Input: dimensioned drawing with shaded views. Units: mm. Origin: part minimum x, y, z. Round coordinates to 2 decimals unless told otherwise and drop trailing zeros. Order: outer loops, then holes, each group sorted by start corner. A loop starts at its lowest first (then second) coordinate and runs counter-clockwise, first axis right, second up. Notation, with made-up numbers: M 17,-8 L 56,-8 A24 ccw 56,23 Z; hole C 80.25,21.25 d9. An arc over 180 degrees is marked long. Put each result on its own line as item: value. Start each with the question number.
1) Section B-B, the plane y = 5.75. Return loops of the section in (x, z) (3 decimals).
2) First-contact query: P1, Ø3, axis at x = 2.5, z = 2.75, coming from the +Y side; P2, Ø5, axis at y = 12, z = 11, coming from the +X side; P3, Ø5, axis at x = 55.5, y = 10, coming from the -Z side. Flat tips, straight axial feed; report the tip coordinate or a pass-through.
3) Section A-A, the plane z = 9. Return loops of the section in (x, y) (3 decimals), then the cut area to 3 significant figures.
4) Section C-C, the plane x = 2.5. Return loops of the section in (y, z) (3 decimals).
5) Material intervals for probe 1 along X at (y, z) = (0.5, 2.75) (3 decimals); probe 2 along Z at (x, y) = (46.5, 0.95) (3 decimals); probe 3 along Y at (x, z) = (31.5, 6), sorted ascending. Write a range as [from, to].
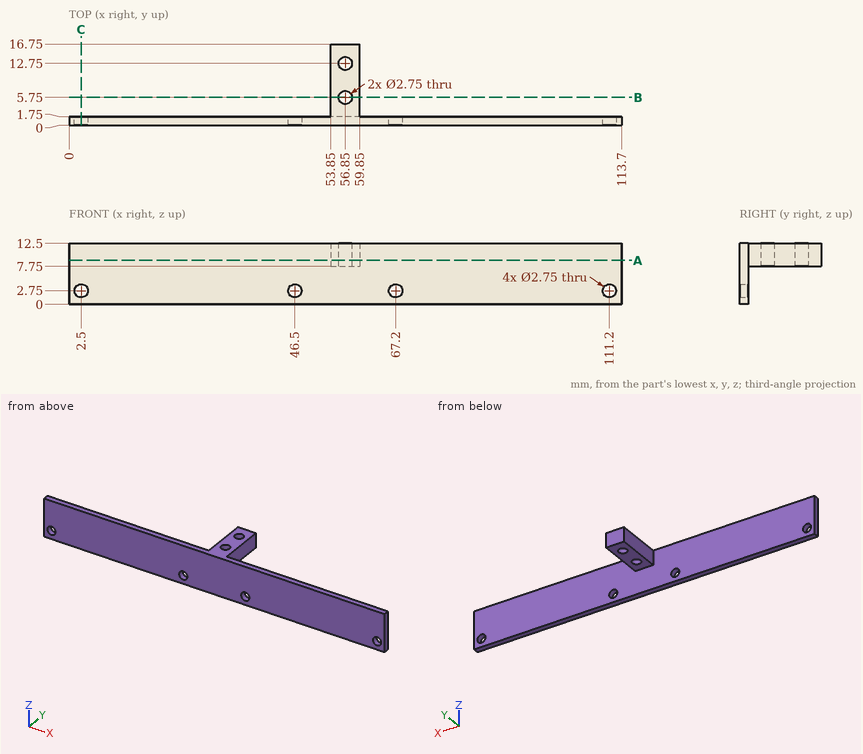
Result sheet:
1. outline: M 53.85,7.75 L 55.475,7.75 L 55.475,12.5 L 53.85,12.5 Z; M 58.225,7.75 L 59.85,7.75 L 59.85,12.5 L 58.225,12.5 Z
2. P1: stops at y = 1.75
2. P2: stops at x = 59.85
2. P3: stops at z = 7.75
3. outline: M 0,0 L 113.7,0 L 113.7,1.75 L 59.85,1.75 L 59.85,16.75 L 53.85,16.75 L 53.85,1.75 L 0,1.75 Z; hole C 56.85,5.75 d2.75; hole C 56.85,12.75 d2.75
3. area: 277 mm2
4. outline: M 0,0 L 1.75,0 L 1.75,1.375 L 0,1.375 Z; M 0,4.125 L 1.75,4.125 L 1.75,12.5 L 0,12.5 Z
5. probe 1: x = [0, 1.125], [3.875, 45.125], [47.875, 65.825], [68.575, 109.825], [112.575, 113.7]
5. probe 2: z = [0, 1.375], [4.125, 12.5]
5. probe 3: y = [0, 1.75]
